```python
from build123d import *

# Parameters (mm, degrees)
F2_DEPTH       = 5
F3_D           = 4.5
F3_CSINK_D     = 8.5
F3_CSINK_ANGLE = 90
F4_R           = 8


with BuildPart() as f2:
    # F1 (on Top) → F2 (new body)
    with BuildSketch(Plane.XY):
        Polygon((36, 35), (-36, 35), (-36, 15), (-16, 15), (-16, -15), (-36, -15), (-36, -35), (36, -35), (36, -15), (16, -15), (16, 15), (36, 15), align=None)
        with BuildLine():
            ThreePointArc((-16, -21.75), (-13.701903, -22.701903), (-12.75, -25))
            ThreePointArc((-12.75, -25), (-13.701903, -27.298097), (-16, -28.25))
            Line((-16, -28.25), (-28, -28.25))
            ThreePointArc((-28, -28.25), (-31.25, -25), (-28, -21.75))
            Line((-28, -21.75), (-16, -21.75))
        make_face(mode=Mode.SUBTRACT)
        with BuildLine():
            ThreePointArc((16, -28.25), (12.75, -25), (16, -21.75))
            Line((16, -21.75), (28, -21.75))
            ThreePointArc((28, -21.75), (30.298097, -22.701903), (31.25, -25))
            ThreePointArc((31.25, -25), (30.298097, -27.298097), (28, -28.25))
            Line((28, -28.25), (16, -28.25))
        make_face(mode=Mode.SUBTRACT)
        with BuildLine():
            ThreePointArc((-16, 28.25), (-13.701903, 27.298097), (-12.75, 25))
            ThreePointArc((-12.75, 25), (-13.701903, 22.701903), (-16, 21.75))
            Line((-16, 21.75), (-28, 21.75))
            ThreePointArc((-28, 21.75), (-31.25, 25), (-28, 28.25))
            Line((-28, 28.25), (-16, 28.25))
        make_face(mode=Mode.SUBTRACT)
        with BuildLine():
            ThreePointArc((16, 21.75), (12.75, 25), (16, 28.25))
            Line((16, 28.25), (28, 28.25))
            ThreePointArc((28, 28.25), (30.298097, 27.298097), (31.25, 25))
            ThreePointArc((31.25, 25), (30.298097, 22.701903), (28, 21.75))
            Line((28, 21.75), (16, 21.75))
        make_face(mode=Mode.SUBTRACT)
    extrude(amount=F2_DEPTH)

    # F3 (through all)
    with Locations(Plane(origin=(0, 0, 0), x_dir=(1, 0, 0), z_dir=(0, 0, -1))):
        with Locations((0, 25), (0, 0), (0, -25)):
            CounterSinkHole(F3_D / 2, F3_CSINK_D / 2, counter_sink_angle=F3_CSINK_ANGLE)

    # F4
    f4_edges = [f2.edges().sort_by_distance(p)[0] for p in [
        (-36, 35, 2.5),
        (-36, -15, 2.5),
        (-36, -35, 2.5),
        (36, -15, 2.5),
        (36, -35, 2.5),
        (36, 15, 2.5),
        (36, 35, 2.5),
        (-16, -15, 2.5),
        (-16, 15, 2.5),
        (16, 15, 2.5),
        (16, -15, 2.5),
        (-36, 15, 2.5),
    ]]
    fillet(f4_edges, radius=F4_R)


solid = f2.part
```
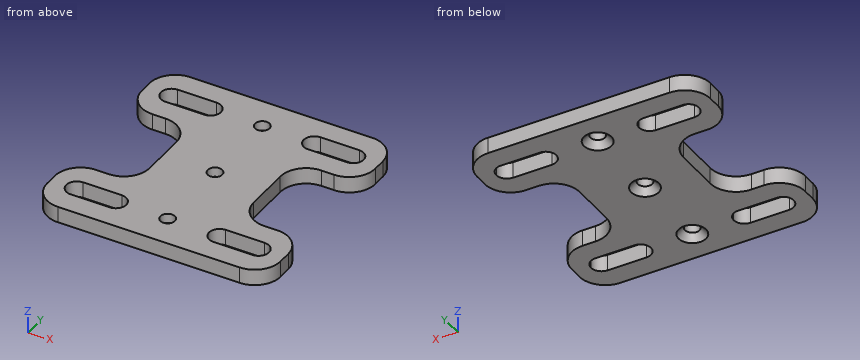
Here's how the part is built. I have some questions about the finished solid (model axes, mm). Round coordinates to 2 decimals unless told otherwise and drop trailing zeros. Order: outer loops, then holes, each group sorted by start corner. A loop starts at its lowest first (then second) coordinate and runs counter-clockwise, first axis right, second up. Notation, with made-up numbers: (7.25, 80.5) -> (46.25, 80.5) arc R11 cw to (46.25, 90.5) -> close; hole circle Ø2 at (13, 86.5). An arc over 180 degrees is marked (long way). Use a Markdown table: item, result. Add a question column.
(1) Suppose I cut it at A-A, the plane x = 0. Please give me the cut outline in (y, z), and give its area (4 significant figures).
(2) Suppose I cut it at D-D, the plane x = 20.5. Please give me the cut outline in (y, z), and give its area (3 significant figures).
(3) Suppose I cut it at B-B, the plane y = 0. Please give me the cut outline in (x, z).
(4) I need wall thicknesses on line 1 along X through (y, z) = (25, 2.8); line 2 along Y through (x, z) = (0, 4.1); line 3 along Y through (x, z) = (-27.5, 3.65). Which ranges of each line are inside material? Lowest first, please.
(5) For pin 1 Ø3 at (y, z) = (-1.5, 1) entering from -X; pin 2 Ø2 at (y, z) = (8, 1) entering from -X; pin 3 Ø2 at (x, y) = (27.5, -13.5) entering from -Z, each with a flat end and sliding along its axis, tell me the tip position at first contact or that it passes through.
(6) Suppose I cut it at C-C, the plane z = 3.4. Count the separate pieces of the cut face and the enclosed holes in it, and give its area (3 significant figures).
Verdict:
| question | item | result |
|---|---|---|
| 1 | outline | (-35, 0) -> (-29.25, 0) -> (-27.25, 2) -> (-27.25, 5) -> (-35, 5) -> close; (-22.75, 2) -> (-20.75, 0) -> (-4.25, 0) -> (-2.25, 2) -> (-2.25, 5) -> (-22.75, 5) -> close; (2.25, 2) -> (4.25, 0) -> (20.75, 0) -> (22.75, 2) -> (22.75, 5) -> (2.25, 5) -> close; (27.25, 2) -> (29.25, 0) -> (35, 0) -> (35, 5) -> (27.25, 5) -> close |
| 1 | area | 270.5 mm2 |
| 2 | outline | (-35, 0) -> (-28.25, 0) -> (-28.25, 5) -> (-35, 5) -> close; (-21.75, 0) -> (-14.19, 0) -> (-14.19, 5) -> (-21.75, 5) -> close; (14.19, 0) -> (21.75, 0) -> (21.75, 5) -> (14.19, 5) -> close; (28.25, 0) -> (35, 0) -> (35, 5) -> (28.25, 5) -> close |
| 2 | area | 143 mm2 |
| 3 | outline | (-16, 0) -> (-4.25, 0) -> (-2.25, 2) -> (-2.25, 5) -> (-16, 5) -> close; (2.25, 2) -> (4.25, 0) -> (16, 0) -> (16, 5) -> (2.25, 5) -> close |
| 4 | line 1 | -36 to -31.25, -12.75 to -2.25, 2.25 to 12.75, 31.25 to 36 |
| 4 | line 2 | -35 to -27.25, -22.75 to -2.25, 2.25 to 22.75, 27.25 to 35 |
| 4 | line 3 | -35 to -28.25, -21.75 to -15, 15 to 21.75, 28.25 to 35 |
| 5 | pin 1 | x = -16 |
| 5 | pin 2 | x = -16.25 |
| 5 | pin 3 | through |
| 6 | separate pieces | 1 |
| 6 | enclosed holes | 7 |
| 6 | area | 3,290 mm2 |
